Geometry: final body of the model. Coordinates: model frame, mm. A direction names the side the tool comes from. Give positions to 0.01 mm unless a question says otherwise; leave off trailing zeros. Write each loop counter-clockwise with the first axis right and the second up, starting at its lowest first coordinate (ties: lowest second). Pieces come first, ordered by that corner, then holes. Notation, with made-up numbers: M 35.5,79.5 L 55.5,79.5 A17 ccw 55.5,92.5 Z; hole C 40,67 d1. An arc over 180 degrees is marked long. Use one line per item in the form item = value. Start each with the question number.
Item 1: Section query A-A on z = 145. Return loops of the section in (x, y).
Item 2: Section query D-D on z = -39. Return loops of the section in (x, y).
Item 3: Access query for faces 5 (the flat face through (0.28, -248.158, 421.338)), 6 (the flat face through (0.28, -335.56, 155.99)). Directions: +Z, -Z, +X, -X, +Y, -Y. A direction counts if a zero-diameter tool reaches every point of the face in a straight line with its end or side. Return the directions, or none.
Item 4: Section query B-B on z = 250. Give the number of separate pieces and of enclosed holes in the cut face, then the cut area to 3 significant figures.
Item 5: Section query C-C on y = 710. Return loops of the section in (x, z).
Item 6: Pull-direction query (Y, two-part tool) for faces 1 (the cylindrical face through (3.15, 340.003, 521.204)), 2 (the flat face through (-20, -143, 102)), 3 (the flat face through (0.28, -28.243, -17.013)), 4 (the flat face through (0.28, -46.14, 22.514)); classes: released by +Y, released by -Y, zero draft, split by the parting line, or undercut.
Item 7: Material intervals for line 1 along X through (y, z) = (212.5, -24); line 2 along Z through (x, y) = (4, 158); line 3 along Y through (x, z) = (-162, 478), sorted ascending. Write a range as from..to.
Item 8: Contact query for flat-ended pins moving along their axis: P1, Ø1.5, axis at y = 467.5, z = 300.5, coming from the +X side; P2, Ø10, axis at y = 227.5, z = 13.5, coming from the -X side. Output: stop coordinate, or through.
from build123d import *

# Parameters (mm, degrees)
F3_DEPTH = 20
F1_R     = 355.6
F1_R_2   = 273.05
F4_DEPTH = 20
F5_R     = 25.4
F6_DEPTH = 225


with BuildPart() as f3:
    # F2 (on Right) → F3 (new body, symmetric)
    with BuildSketch(Plane.YZ):
        with BuildLine():
            Line((539.424256, 38.240109), (338.68509, 519.698787))
            Line((338.68509, 519.698787), (-218.144057, 482.688492))
            Line((-218.144057, 482.688492), (-447.444623, 13.987639))
            Line((-447.444623, 13.987639), (9.804998, -19.827125))
            Line((9.804998, -19.827125), (322.617488, 459.231032))
            Line((322.617488, 459.231032), (504.258433, 23.578087))
            ThreePointArc((504.258433, 23.578087), (529.172356, 13.326186), (539.424256, 38.240109))
        make_face()
        Polygon((-388.472688, 47.830557), (-206.728306, 419.324393), (-30.299405, 21.342738), align=None, mode=Mode.SUBTRACT)
        Polygon((0, 47.005516), (-181.525694, 456.484325), (287.745681, 487.674991), align=None, mode=Mode.SUBTRACT)
    extrude(amount=F3_DEPTH, both=True)

    # F1 (on Right) → F4 (join, symmetric)
    with BuildSketch(Plane.YZ):
        with Locations((-417.958655, 30.909098)):
            Circle(F1_R)
        with Locations((-417.958655, 30.909098)):
            Circle(F1_R_2, mode=Mode.SUBTRACT)
        with Locations((521.841345, 30.909098)):
            Circle(F1_R)
        with Locations((521.841345, 30.909098)):
            Circle(F1_R_2, mode=Mode.SUBTRACT)
    extrude(amount=F4_DEPTH, both=True)

    # F5 (on Right) → F6 (join, symmetric)
    with BuildSketch(Plane.YZ):
        with Locations((326.347711, 499.786736)):
            Circle(F5_R)
    extrude(amount=F6_DEPTH, both=True)


solid = f3.part
Answer sheet:
q1.outline = M -20,-754.76 L 20,-754.76 L 20,-666.03 L -20,-666.03 Z; M -20,-383.35 L 20,-383.35 L 20,-340.93 L -20,-340.93 Z; M -20,-169.89 L 20,-169.89 L 20,-43.44 L -20,-43.44 Z; M -20,63.99 L 20,63.99 L 20,117.43 L -20,117.43 Z; M -20,185.04 L 20,185.04 L 20,273.77 L -20,273.77 Z; M -20,453.63 L 20,453.63 L 20,494.91 L -20,494.91 Z; M -20,769.91 L 20,769.91 L 20,858.64 L -20,858.64 Z
q2.outline = M -20,-766.62 L 20,-766.62 L 20,-681.91 L -20,-681.91 Z; M -20,-154.01 L 20,-154.01 L 20,-69.3 L -20,-69.3 Z; M -20,173.18 L 20,173.18 L 20,257.89 L -20,257.89 Z; M -20,785.79 L 20,785.79 L 20,870.5 L -20,870.5 Z
q3.face_5 = +Z, +X, -X
q3.face_6 = +X, -X
q4.separate_pieces = 8
q4.enclosed_holes = 0
q4.area = 25,900 mm2
q5.outline = M -20,-270.83 L 20,-270.83 L 20,-166.96 L -20,-166.96 Z; M -20,228.78 L 20,228.78 L 20,332.65 L -20,332.65 Z
q6.face_1 = split by the parting line
q6.face_2 = zero draft
q6.face_3 = undercut
q6.face_4 = undercut
q7.line_1 = -20..20
q7.line_2 = 207.13..288.98, 479.05..507.69
q7.line_3 = 313.29..339.41
q8.P1 = 20
q8.P2 = -20
